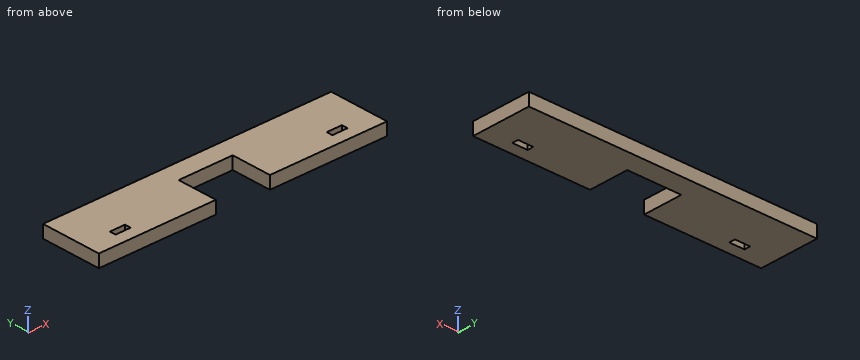
```python
from build123d import *

# Parameters (mm, degrees)
SKETCH1_W           = 3.81
SKETCH1_H           = 1.524
BOSS_EXTRUDE1_DEPTH = 3.1115


with BuildPart() as part:
    # Sketch1 → Boss-Extrude1 (new body)
    with BuildSketch(Plane.XY):
        Polygon((-36.017419718, -7.591435707), (-6.767419718, -7.591435707), (-6.767419718, 2.408564293), (6.732580282, 2.408564293), (6.732580282, -7.591435707), (35.982580282, -7.591435707), (35.982580282, -5.091435707), (35.982580282, 4.908564293), (35.982580282, 7.408564293), (-36.017419718, 7.408564293), (-36.017419718, 4.908564293), (-36.017419718, -5.091435707), align=None)
        with Locations((27.077580282, -3.781435707)):
            Rectangle(SKETCH1_W, SKETCH1_H, mode=Mode.SUBTRACT)
        with Locations((-27.112419718, -3.781435707)):
            Rectangle(SKETCH1_W, SKETCH1_H, mode=Mode.SUBTRACT)
    extrude(amount=BOSS_EXTRUDE1_DEPTH)


solid = part.part
```
Can you work these out from the model? Positions are in its coordinate system, mm. Coordinates: 2 decimals unless noted, no trailing zeros. Loops run counter-clockwise (first coordinate to the right, second up) from the corner with the lowest first, then second, coordinate; pieces in that order, holes last. Notation, with made-up numbers: M 63.25,-10 L 89.25,-10 A24 ccw 89.25,12 Z; hole C -34,51 d10. An arc over 180 degrees is marked long. Put each result on its own line as item: value. Start each with the question number.
(1) Will this pin go through, and if not, where does the flat tip stop? pin 1 Ø1.6 at (x, z) = (-3, 1) entering from -Y.
(2) Imagine slicing it at C-C on x = -4. List the corners of the cut face in (y, z) for me, and give its area (3 significant figures).
(3) Imagine slicing it at B-B on z = 2.2. List the corners of the cut face in (x, y) for me.
(4) I need wall thicknesses on probe 1 along X at (y, z) = (-4.5, 2.05); probe 2 along X at (y, z) = (-0.5, 0.8); probe 3 along Y at (x, z) = (28.5, 2.1). Which ranges of each line are inside material? Lowest first, please.
(5) Imagine slicing it at A-A on y = -0.25. List the corners of the cut face in (x, z) for me, and give its area (3 significant figures).
Worked answers:
1. pin 1: stops at y = 2.41
2. outline: M 2.41,0 L 7.41,0 L 7.41,3.11 L 2.41,3.11 Z
2. area: 15.6 mm2
3. outline: M -36.02,-7.59 L -6.77,-7.59 L -6.77,2.41 L 6.73,2.41 L 6.73,-7.59 L 35.98,-7.59 L 35.98,7.41 L -36.02,7.41 Z; hole M -29.02,-4.54 L -25.21,-4.54 L -25.21,-3.02 L -29.02,-3.02 Z; hole M 25.17,-4.54 L 28.98,-4.54 L 28.98,-3.02 L 25.17,-3.02 Z
4. probe 1: x = -36.02 to -29.02, -25.21 to -6.77, 6.73 to 25.17, 28.98 to 35.98
4. probe 2: x = -36.02 to -6.77, 6.73 to 35.98
4. probe 3: y = -7.59 to -4.54, -3.02 to 7.41
5. outline: M -36.02,0 L -6.77,0 L -6.77,3.11 L -36.02,3.11 Z; M 6.73,0 L 35.98,0 L 35.98,3.11 L 6.73,3.11 Z
5. area: 182 mm2
